Work out the finished part from the listing and answer in its coordinate system (mm). A direction names the side the tool comes from. Give positions to 0.01 mm unless a question says otherwise; leave off trailing zeros. Loops run counter-clockwise (first coordinate to the right, second up) from the corner with the lowest first, then second, coordinate; pieces in that order, holes last. Notation, with made-up numbers: M 27.25,-26.5 L 45.25,-26.5 A21 ccw 45.25,4.5 Z; hole C 54,-14 d6. An arc over 180 degrees is marked long. Answer as a JSON object with one key per item and string values. Group by question number.
```python
from build123d import *

# Parameters (mm, degrees)
SKETCH1_W               = 15
SKETCH1_H               = 3.75
BOSS_EXTRUDE1_DEPTH     = 7.5
SKETCH2_W               = 15
SKETCH2_H               = 3.75
BOSS_EXTRUDE2_DEPTH     = 15
SKETCH3_R               = 1.6
CUT_EXTRUDE1_DEPTH      = 20.931523399
CUT_EXTRUDE1_DEPTH_BACK = 3.75


with BuildPart() as part:
    # Sketch1 → Boss-Extrude1 (new body)
    with BuildSketch(Plane.XY):
        Rectangle(SKETCH1_W, SKETCH1_H)
    extrude(amount=BOSS_EXTRUDE1_DEPTH)

    # Sketch2 → Boss-Extrude2 (add)
    with BuildSketch(Plane(origin=(0, 1.875, 0), x_dir=(1, 0, 0), z_dir=(0, 1, 0))):
        with Locations((0, -5.625)):
            Rectangle(SKETCH2_W, SKETCH2_H)
    extrude(amount=BOSS_EXTRUDE2_DEPTH)

    # Sketch3 → Cut-Extrude1 (cut, two sides)
    with BuildSketch(Plane.XY.offset(7.5)) as cut_extrude1_sk:
        with Locations((0, 9.375)):
            Circle(SKETCH3_R)
        with BuildLine():
            ThreePointArc((-3e-08, 16.875), (5.303300848, 14.67830087), (7.5, 9.375))
            Line((7.5, 9.375), (7.5, 16.875))
            Line((7.5, 16.875), (-3e-08, 16.875))
        make_face()
        with BuildLine():
            ThreePointArc((-7.5, 9.375), (-5.30330087, 14.678300848), (-3e-08, 16.875))
            Line((-3e-08, 16.875), (-7.5, 16.875))
            Line((-7.5, 16.875), (-7.5, 9.375))
        make_face()
    extrude(amount=CUT_EXTRUDE1_DEPTH, mode=Mode.SUBTRACT)
    extrude(cut_extrude1_sk.sketch, amount=-CUT_EXTRUDE1_DEPTH_BACK, mode=Mode.SUBTRACT)

    # Mirror1: part across plane


with BuildPart() as part_1:
    add(part.part)
    add(part.part.mirror(Plane(origin=(0, 0, 0), x_dir=(1, 0, 0), z_dir=(0, 0, -1))))


solid = part_1.part
```
Item 1: Given pin 1 Ø3 at (y, z) = (11.5, -3.5) entering from +X; pin 2 Ø5 at (y, z) = (14, -5.5) entering from -X; pin 3 Ø6 at (x, z) = (-3.5, 0.5) entering from +Y (3 decimals), each flat-ended and moving along its own axis, determine where each tip first touches the part or whether it passes through.
Item 2: A tool of negligible diameter and unlimited length cuts with its end or side. For faces 1 (the flat face through (-0.1, 7.6, -3.75)), 2 (the flat face through (0, -1.875, 0)), from which of +Z, -Z, +X, -X, +Y, -Y can it reach the whole face along a straight path? Write none if from no direction.
Item 3: A cutting plane is placed at A-A (z = 4). Determine the outline of the cut face in (x, y) (3 decimals), and give its area (3 significant figures).
Item 4: A cutting plane is placed at C-C (x = -0.25). Determine the outline of the cut face in (y, z) (3 decimals).
Item 5: Find the intervals of material crossed by probe 1 along Z at (x, y) = (-1.5, 16.25); probe 2 along Y at (x, z) = (0, 5.9) (3 decimals); probe 3 along Y at (x, z) = (-1, -4.5) (3 decimals), in increasing order. Write a range as [from, to].
Item 6: For a pull along Z with two mould halves and no side action, classify faces 3 (the flat face through (-0.1, 7.6, 3.75)), 4 (the flat face through (0, 7, 7.5)), 5 (the cylindrical face through (-0.347, 7.813, -5.651)), 6 (the flat face through (0, 1.875, 0)) as pulls with the +Z half, pulls with the -Z half, needs draft (parallel to the pull), parting line crosses it, or undercut.
Item 7: A cutting plane is placed at B-B (y = 2.5). Determine the outline of the cut face in (x, z), and give its area (4 significant figures).
Item 8: A cutting plane is placed at D-D (x = -6). Determine the outline of the cut face in (y, z) (3 decimals).
The answers:
{
 "1": {"pin 1": "stops at x = 7.47", "pin 2": "stops at x = -7.19", "pin 3": "stops at y = 1.875"},
 "2": {"face 1": "+X, -X, +Y", "face 2": "+Z, -Z, +X, -X, -Y"},
 "3": {"outline": "M -7.5,-1.875 L 7.5,-1.875 L 7.5,9.375 A7.5 ccw -7.5,9.375 Z; hole C 0,9.375 d3.2", "area": "249 mm^2"},
 "4": {"outline": "M -1.875,-7.5 L 7.795,-7.5 L 7.795,-3.75 L 1.875,-3.75 L 1.875,3.75 L 7.795,3.75 L 7.795,7.5 L -1.875,7.5 Z; M 10.955,-7.5 L 16.871,-7.5 L 16.871,-3.75 L 10.955,-3.75 Z; M 10.955,3.75 L 16.871,3.75 L 16.871,7.5 L 10.955,7.5 Z"},
 "5": {"probe 1": "z = [-7.5, -3.75], [3.75, 7.5]", "probe 2": "y = [-1.875, 7.775], [10.975, 16.875]", "probe 3": "y = [-1.875, 8.126], [10.624, 16.808]"},
 "6": {"face 3": "undercut", "face 4": "pulls with the +Z half", "face 5": "needs draft", "face 6": "undercut"},
 "7": {"outline": "M -7.5,-7.5 L 7.5,-7.5 L 7.5,-3.75 L -7.5,-3.75 Z; M -7.5,3.75 L 7.5,3.75 L 7.5,7.5 L -7.5,7.5 Z", "area": "112.5 mm^2"},
 "8": {"outline": "M -1.875,-7.5 L 13.875,-7.5 L 13.875,-3.75 L 1.875,-3.75 L 1.875,3.75 L 13.875,3.75 L 13.875,7.5 L -1.875,7.5 Z"}
}
